Could you check a few things on this model? Use its own coordinates, in mm. Coordinates: 2 decimals unless noted, no trailing zeros. Loops run counter-clockwise (first coordinate to the right, second up) from the corner with the lowest first, then second, coordinate; pieces in that order, holes last.
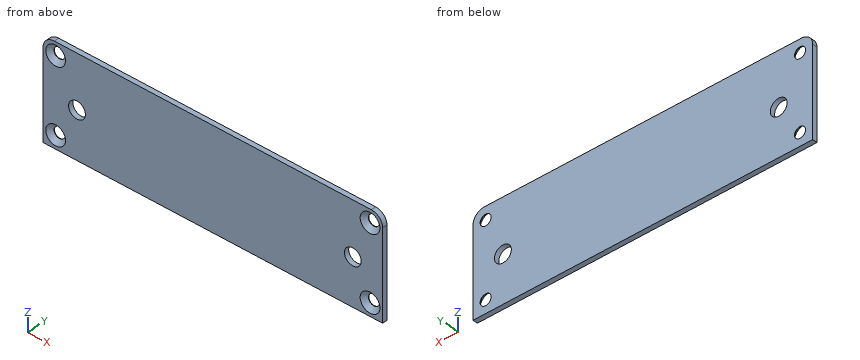
from build123d import *

# Parameters (mm, degrees)
SKETCH_W            = 104.8
SKETCH_H            = 31
PAD_DEPTH           = 1.5
HOLE_D              = 3.4
HOLE_DEPTH          = 25
HOLE_CSINK_D        = 6.1
HOLE_CSINK_ANGLE    = 90
FILLET_R            = 3.5
SKETCH002_R         = 2.6
POCKET_DEPTH        = 1.501
LINEARPATTERN_COUNT = 2
LINEARPATTERN_PITCH = 85.09


with BuildPart() as part:
    # Sketch → Pad (new body)
    with BuildSketch(Plane.XZ):
        Rectangle(SKETCH_W, SKETCH_H)
    extrude(amount=PAD_DEPTH)

    # Hole
    with Locations(Plane.XZ.offset(1.5)):
        with Locations((-48.5, 11.5), (-48.5, -11.5), (48.5, -11.5), (48.5, 11.5)):
            CounterSinkHole(HOLE_D / 2, HOLE_CSINK_D / 2, depth=HOLE_DEPTH, counter_sink_angle=HOLE_CSINK_ANGLE)

    # Fillet
    fillet_edges = [part.edges().sort_by_distance(p)[0] for p in [
        (-52.4, -0.75, 15.5),
        (52.4, -0.75, 15.5),
    ]]
    fillet(fillet_edges, radius=FILLET_R)

    # Sketch002 (on Face5 of Fillet) → Pocket (cut, through all)
    with BuildSketch(Plane.XZ.offset(1.5)):
        with Locations((-41.91, -0.94)):
            Circle(SKETCH002_R)
    pocket = extrude(amount=-POCKET_DEPTH, mode=Mode.SUBTRACT)

    # LinearPattern: Pocket ×2
    with Locations(*[(i * LINEARPATTERN_PITCH, 0, 0) for i in range(1, LINEARPATTERN_COUNT)]):
        add(pocket, mode=Mode.SUBTRACT)


solid = part.part
(1) Imagine slicing it at B-B, the plane y = -1.1. Write out the boundary of the cut face in (x, z).
Answers:
outline: (-52.4, -15.5) - (52.4, -15.5) - (52.4, 12) arc R3.5 ccw to (48.9, 15.5) - (-48.9, 15.5) arc R3.5 ccw to (-52.4, 12) - close; hole circle Ø5.3 at (-48.5, -11.5); hole circle Ø5.3 at (-48.5, 11.5); hole circle Ø5.2 at (-41.91, -0.94); hole circle Ø5.2 at (43.18, -0.94); hole circle Ø5.3 at (48.5, -11.5); hole circle Ø5.3 at (48.5, 11.5)
(2) For pin 1 (4.5 mm diameter, centred on x = -48.5, z = 11.5, fed in from -Y), with a flat end and sliding along its axis, tell me the tip position at first contact or that it passes through.
Answers:
pin 1: stops at y = -0.7
(3) I need wall thicknesses on probe 1 along X at (y, z) = (-0.1, -11.5); probe 2 along Z at (x, y) = (48.5, -0.1); probe 3 along Z at (x, y) = (43.18, -0.65). Which ranges of each line are inside material? Lowest first, please.
Answers:
probe 1: x = -52.4 to -50.2, -46.8 to 46.8, 50.2 to 52.4
probe 2: z = -15.5 to -13.2, -9.8 to 9.8, 13.2 to 15.5
probe 3: z = -15.5 to -3.54, 1.66 to 15.5
(4) Imagine slicing it at C-C, the plane z = -11.5. Write out the boundary of the cut face in (x, y), and give its area (3 significant figures).
Answers:
outline: (-52.4, -1.5) - (-51.55, -1.5) - (-50.2, -0.15) - (-50.2, 0) - (-52.4, 0) - close; (-46.8, -0.15) - (-45.45, -1.5) - (45.45, -1.5) - (46.8, -0.15) - (46.8, 0) - (-46.8, 0) - close; (50.2, -0.15) - (51.55, -1.5) - (52.4, -1.5) - (52.4, 0) - (50.2, 0) - close
area: 143 mm2
(5) Imagine slicing it at A-A, the plane z = -2.5. Write out the boundary of the cut face in (x, y), and give its area (3 significant figures).
Answers:
outline: (-52.4, -1.5) - (-43.99, -1.5) - (-43.99, 0) - (-52.4, 0) - close; (-39.83, -1.5) - (41.1, -1.5) - (41.1, 0) - (-39.83, 0) - close; (45.26, -1.5) - (52.4, -1.5) - (52.4, 0) - (45.26, 0) - close
area: 145 mm2
